Design review of the part built by this model. Coordinates are the model's own, in mm. Round coordinates to 2 decimals unless told otherwise and drop trailing zeros. Loops run counter-clockwise (first coordinate to the right, second up) from the corner with the lowest first, then second, coordinate; pieces in that order, holes last. Notation, with made-up numbers: M 28.5,-12 L 50.5,-12 A19 ccw 50.5,3 Z; hole C -28,51.5 d9. An arc over 180 degrees is marked long. Use a Markdown table: item, result.
from build123d import *

# Parameters (mm, degrees)
F1_DEPTH = 2.5
F2_R     = 5
F3_R     = 5


with BuildPart() as f1:
    # F0 (on Front) → F1 (new body)
    with BuildSketch(Plane.XZ):
        Polygon((9.486825, 28.460502), (-19.904105, 22.446082), (-29.39093, -6.014419), (-9.486825, -28.460502), (19.904105, -22.446082), (29.39093, 6.014419), align=None)
        Polygon((-16.586754, 18.705069), (7.905688, 23.717085), (24.492442, 5.012016), (16.586754, -18.705069), (-7.905688, -23.717085), (-24.492442, -5.012016), align=None, mode=Mode.SUBTRACT)
    extrude(amount=F1_DEPTH)

    # F2
    f2_edges = [f1.edges().sort_by_distance(p)[0] for p in [
        (-19.904105, -1.25, 22.446082),
        (9.486825, -1.25, 28.460502),
        (29.39093, -1.25, 6.014419),
        (19.904105, -1.25, -22.446082),
        (-9.486825, -1.25, -28.460502),
        (-29.39093, -1.25, -6.014419),
    ]]
    fillet(f2_edges, radius=F2_R)

    # F3
    f3_edges = [f1.edges().sort_by_distance(p)[0] for p in [
        (-24.492442, -1.25, -5.012016),
        (-7.905688, -1.25, -23.717085),
        (16.586754, -1.25, -18.705069),
        (7.905688, -1.25, 23.717085),
        (-16.586754, -1.25, 18.705069),
    ]]
    fillet(f3_edges, radius=F3_R)


solid = f1.part
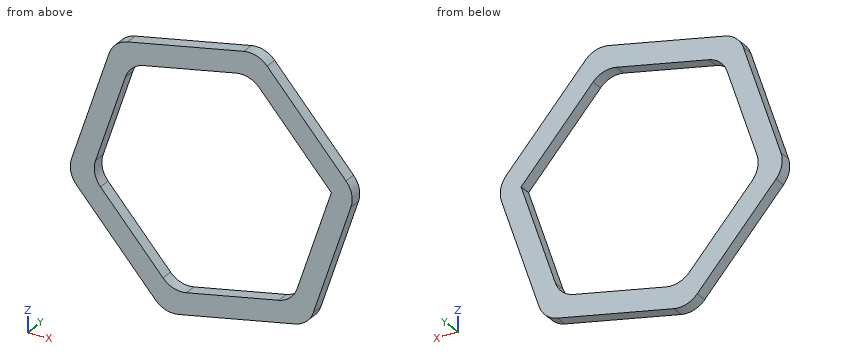
1. Take a section at A-A on y = -1.55. Give the boundary of the cut face in (x, z), and give its area (3 significant figures).
Check values:
| item | result |
|---|---|
| outline | M -28.48,-3.28 A5 ccw -27.48,-8.17 L -11.4,-26.3 A5 ccw -6.66,-27.88 L 17.08,-23.02 A5 ccw 20.82,-19.71 L 28.48,3.28 A5 ccw 27.48,8.17 L 11.4,26.3 A5 ccw 6.66,27.88 L -17.08,23.02 A5 ccw -20.82,19.71 Z; hole M -23.58,-2.27 A5 ccw -22.58,-7.17 L -9.82,-21.56 A5 ccw -5.08,-23.14 L 13.76,-19.28 A5 ccw 17.5,-15.97 L 24.49,5.01 L 9.82,21.56 A5 ccw 5.08,23.14 L -13.76,19.28 A5 ccw -17.5,15.97 Z |
| area | 713 mm² |
2. Insertion check: pin 1 (8 mm diameter, centred on x = -0.5, z = -21, fed in from -Y); pin 2 (1 mm diameter, centred on x = -16, y = -2, fed in from -Z). Each pin has a flat end and moves straight along its axis. Give the tip position at first contact, or say it passes through.
Check values:
| item | result |
|---|---|
| pin 1 | stops at y = -2.5 |
| pin 2 | stops at z = -21.68 |
3. Wall thickness on line 1 along Z through (x, y) = (-3.5, -1.55); line 2 along X through (y, z) = (-1.35, -7); line 3 along Z through (x, y) = (6.5, -0.5): over which ranges is each line inside the solid? List them lowest first. Write a range as from..to.
Check values:
| item | result |
|---|---|
| line 1 | z = -27.24..-22.82, 21.38..25.8 |
| line 2 | x = -28.25..-22.72, 20.49..25.05 |
| line 3 | z = -25.19..-20.77, 23.22..27.85 |
4. Take a section at D-D on x = -25. Give the boundary of the cut face in (y, z).
Check values:
| item | result |
|---|---|
| outline | M -2.5,-10.97 L 0,-10.97 L 0,7.16 L -2.5,7.16 Z |
5. Take a section at B-B on z = -1. Give the boundary of the cut face in (x, y), and give its area (3 significant figures).
Check values:
| item | result |
|---|---|
| outline | M -27.72,-2.5 L -23.16,-2.5 L -23.16,0 L -27.72,0 Z; M 22.49,-2.5 L 27.05,-2.5 L 27.05,0 L 22.49,0 Z |
| area | 22.8 mm² |
6. Take a section at C-C on x = -3.5. Give the boundary of the cut face in (y, z), and give its area (3 significant figures).
Check values:
| item | result |
|---|---|
| outline | M -2.5,-27.24 L 0,-27.24 L 0,-22.82 L -2.5,-22.82 Z; M -2.5,21.38 L 0,21.38 L 0,25.8 L -2.5,25.8 Z |
| area | 22.1 mm² |
